Design review of the part shown in the three views and the two pictorial views. Dimensions are in mm from the part's minimum x, y and z. A direction names the side the tool comes from. Give positions to 0.01 mm unless a question says otherwise; leave off trailing zeros. Loops run counter-clockwise (first coordinate to the right, second up) from the corner with the lowest first, then second, coordinate; pieces in that order, holes last. Notation, with made-up numbers: (-23.5, -14) - (18.5, -14) arc R21 cw to (18.5, 4) - close; hole circle Ø8 at (-0.5, 72.5). An arc over 180 degrees is marked (long way). Return JSON: item names as keys, results as strings. Group by question number.
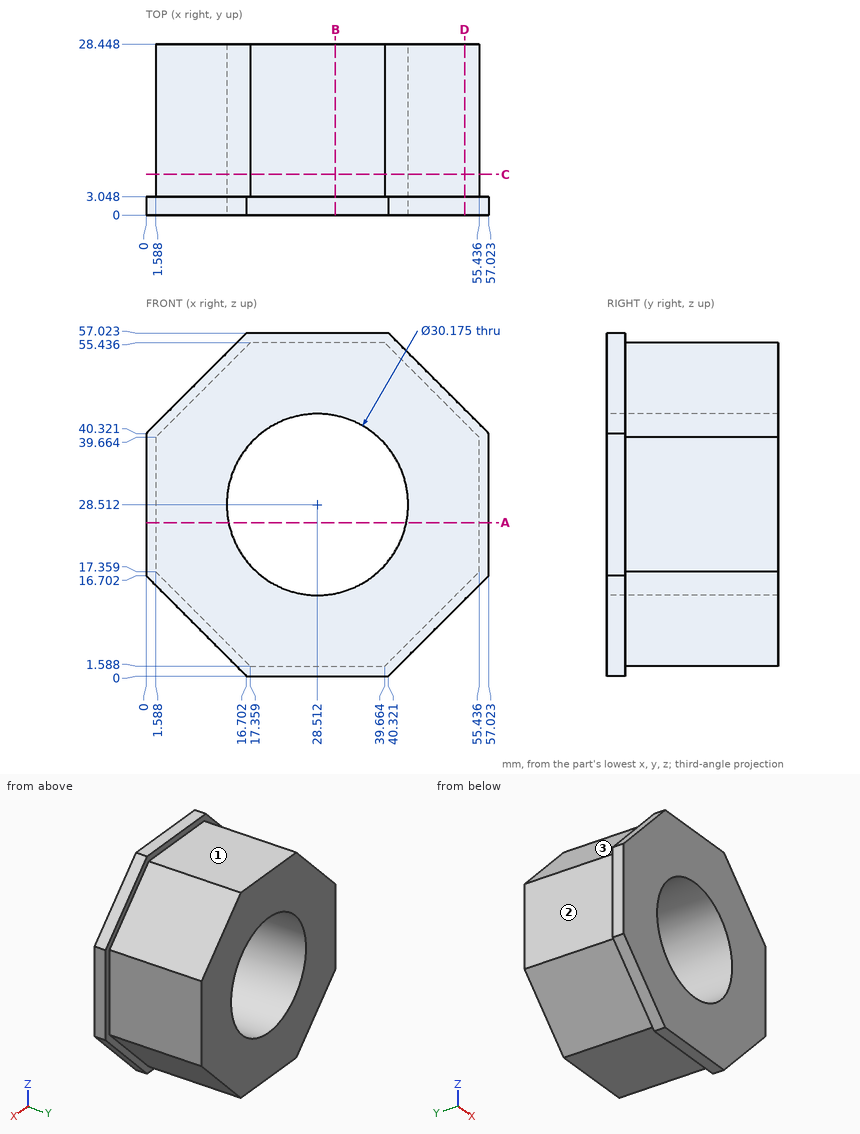
Item 1: For P1, Ø11, axis at x = 27, y = 17, coming from the -Z side; P2, Ø1.5, axis at x = 49, y = 25.5, coming from the +Z side; P3, Ø1, axis at x = 12, y = 9.5, coming from the -Z side (1 decimal), all flat-tipped, find the tip position at first contact; note any pin that passes through.
Item 2: Tool access review of the marked faces 1, 2 and 3: name each direction out of +Z, -Z, +X, -X, +Y, -Y from which nothing blocks a thin tool from reaching the whole face with its end or side.
Item 3: For L1, parallel to Z at x = 32, y = 17.25 (1 decimal); L2, parallel to X at y = 21.75, z = 26.5 (1 decimal); L3, parallel to X at y = 24.5, z = 22 (1 decimal), list the stretches that pass through material, from the lowest coordinate up. Write a range as from..to.
Item 4: Take a section at A-A (z = 25.5). State the section outline as (x, y) points (1 decimal).
Item 5: Take a section at D-D (x = 53). State the section outline as (y, z) points (1 decimal).
Item 6: Take a section at B-B (x = 31.5). State the section outline as (y, z) points (1 decimal), then the cut area to 3 significant figures.
Item 7: Take a section at C-C (y = 6.75). State the section outline as (x, z) points (1 decimal), then the cut area to 3 significant figures.
Check sheet entries:
{
 "1": {"P1": "stops at z = 1.59", "P2": "stops at z = 46.85", "P3": "stops at z = 6.4"},
 "2": {"face 1": "+Z, +X, -X, +Y", "face 2": "+Z, -Z, -X, +Y", "face 3": "+Z, -X, +Y"},
 "3": {"L1": "z = 1.6..13.8, 43.2..55.4", "L2": "x = 1.6..13.6, 43.5..55.4", "L3": "x = 1.6..14.9, 42.1..55.4"},
 "4": {"outline": "(0, 0) - (13.7, 0) - (13.7, 28.4) - (1.6, 28.4) - (1.6, 3) - (0, 3) - close; (43.3, 0) - (57, 0) - (57, 3) - (55.4, 3) - (55.4, 28.4) - (43.3, 28.4) - close"},
 "5": {"outline": "(0, 12.7) - (3, 12.7) - (3, 14.9) - (28.4, 14.9) - (28.4, 42.1) - (3, 42.1) - (3, 44.3) - (0, 44.3) - close"},
 "6": {"outline": "(0, 0) - (3, 0) - (3, 1.6) - (28.4, 1.6) - (28.4, 13.7) - (0, 13.7) - close; (0, 43.3) - (28.4, 43.3) - (28.4, 55.4) - (3, 55.4) - (3, 57) - (0, 57) - close", "area": "700 mm^2"},
 "7": {"outline": "(1.6, 17.4) - (17.4, 1.6) - (39.7, 1.6) - (55.4, 17.4) - (55.4, 39.7) - (39.7, 55.4) - (17.4, 55.4) - (1.6, 39.7) - close; hole circle Ø30.2 at (28.5, 28.5)", "area": "1,690 mm^2"}
}
